For this review, take the finished solid that the model builds, in its own axes (mm). A direction names the side the tool comes from. Coordinates: 2 decimals unless noted, no trailing zeros. Write each loop counter-clockwise with the first axis right and the second up, starting at its lowest first coordinate (ties: lowest second). Pieces come first, ordered by that corner, then holes.
```python
from build123d import *

# Parameters (mm, degrees)
SKETCH1_R           = 10.5
SKETCH1_R_2         = 8
BOSS_EXTRUDE1_DEPTH = 7


with BuildPart() as part:
    # Sketch1 → Boss-Extrude1 (new body)
    with BuildSketch(Plane.XY):
        with BuildLine():
            Line((25.403411844, 18), (40.04634859, 43.362310416))
            ThreePointArc((40.04634859, 43.362310416), (40.729032534, 47.562011618), (38.455388874, 51.158411493))
            ThreePointArc((38.455388874, 51.158411493), (-35.819868425, 53.037128749), (-61.819252882, -16.564418887))
            Line((-61.819252882, -16.564418887), (-60.007519567, -23.325899671))
            ThreePointArc((-60.007519567, -23.325899671), (-57.211964609, -26.969137823), (-52.659050338, -27.568540358))
            Line((-52.659050338, -27.568540358), (-10.79860525, -16.352067901))
            ThreePointArc((-10.79860525, -16.352067901), (-8.844993295, -16.161017697), (-6.934268235, -16.610717144))
            ThreePointArc((-6.934268235, -16.610717144), (4.455015534, -17.439978113), (14.051245496, -11.25))
            ThreePointArc((14.051245496, -11.25), (16.136917784, -9.591673087), (18.734993995, -9))
            Line((18.734993995, -9), (68.906523061, -9))
            ThreePointArc((68.906523061, -9), (71.299695166, -9.497934272), (73.295653135, -10.909090909))
            ThreePointArc((73.295653135, -10.909090909), (101, 0), (73.295653135, 10.909090909))
            ThreePointArc((73.295653135, 10.909090909), (71.299695166, 9.497934272), (68.906523061, 9))
            Line((68.906523061, 9), (30.599564267, 9))
            ThreePointArc((30.599564267, 9), (25.403411844, 12), (25.403411844, 18))
        make_face()
        Circle(SKETCH1_R, mode=Mode.SUBTRACT)
        with Locations((85, 0)):
            Circle(SKETCH1_R_2, mode=Mode.SUBTRACT)
        with BuildLine():
            Line((-22.446087833, -6.014411108), (-43.078559215, -11.542865153))
            ThreePointArc((-43.078559215, -11.542865153), (-47.971955445, -10.731402919), (-50.582336617, -6.513618221))
            ThreePointArc((-50.582336617, -6.513618221), (-31.046832879, 40.461020355), (19.383344125, 47.172936845))
            ThreePointArc((19.383344125, 47.172936845), (22.781794932, 43.559859246), (22.299103121, 38.623179569))
            Line((22.299103121, 38.623179569), (11.618950039, 20.124611797))
            ThreePointArc((11.618950039, 20.124611797), (8.69359949, 17.570923037), (4.817098212, 17.343458848))
            ThreePointArc((4.817098212, 17.343458848), (-10.957705722, 14.280360125), (-17.999251578, -0.164142113))
            ThreePointArc((-17.999251578, -0.164142113), (-19.222277472, -3.849682749), (-22.446087833, -6.014411108))
        make_face(mode=Mode.SUBTRACT)
    extrude(amount=BOSS_EXTRUDE1_DEPTH)


solid = part.part
```
1) Consider section D-D (z = 4.5). Give the boundary of the cut face in (x, y) (3 decimals), then the cut area to 3 significant figures.
2) Tool access review of faces 1 (the face through (50, 9, 3)), 2 (the face through (71.3, -9.5, 3.5)), 3 (the face through (17, 19, 0)): name each direction out of +Z, -Z, +X, -X, +Y, -Y from which nothing blocks a thin tool from reaching the whole face with its end or side.
3) The part is to be moulded in two halves that separate along X. For faces 4 (the face through (-47.91, -10.77, 3.45)), 5 (the face through (-34.895, 53.65, 3.451)), 6 (the face through (40.74, 47.5, 3.45)), say which applies: pulls with the +X half, pulls with the -X half, needs draft (parallel to the pull), parting line crosses it, or undercut.
4) Clearance check with flat-ended pins moving along their axes: P1, Ø4, axis at y = 4, z = 5, coming from the +X side; P2, Ø10, axis at x = -1, y = -14.5, coming from the -Z side; P3, Ø3.5, axis at x = 53, z = 2.5, coming from the +Y side; P4, Ø3.5, axis at x = 53.5, z = 3, coming from the -Y side. State where each tip first meets the part, or that it passes through.
5) Consider section B-B (x = 0). Give the boundary of the cut face in (y, z).
6) Consider section A-A (x = 85). Give the boundary of the cut face in (y, z).
7) Consider section C-C (y = 41.5). Give the boundary of the cut face in (x, z), then the cut area to 3 significant figures.
8) For L1, parallel to Y at x = 0, z = 1.5; L2, parallel to Y at x = -3.5, z = 5.75; L3, parallel to Y at x = 85, z = 5, list the stretches that pass through material, from the lowest coordinate up.
Results:
1. outline: (-61.819, -16.564) - (-60.008, -23.326) arc R6 ccw to (-52.659, -27.569) - (-10.799, -16.352) arc R6 cw to (-6.934, -16.611) arc R18 ccw to (14.051, -11.25) arc R6 cw to (18.735, -9) - (68.907, -9) arc R6 cw to (73.296, -10.909) arc R16 ccw (long way) to (73.296, 10.909) arc R6 cw to (68.907, 9) - (30.6, 9) arc R6 cw to (25.403, 18) - (40.046, 43.362) arc R6 ccw to (38.455, 51.158) arc R64 ccw to start; hole (-50.582, -6.514) arc R6 ccw to (-43.079, -11.543) - (-22.446, -6.014) arc R6 ccw to (-17.999, -0.164) arc R18 cw to (4.817, 17.343) arc R6 ccw to (11.619, 20.125) - (22.299, 38.623) arc R6 ccw to (19.383, 47.173) arc R51 ccw to start; hole circle Ø21 at (0, 0); hole circle Ø16 at (85, 0)
1. area: 5,250 mm2
2. face 1: +Z, -Z
2. face 2: +Z, -Z, -Y
2. face 3: -Z, +X, -X, +Y, -Y
3. face 4: undercut
3. face 5: parting line crosses it
3. face 6: pulls with the +X half
4. P1: stops at x = 100.87
4. P2: stops at z = 0
4. P3: stops at y = 9
4. P4: stops at y = -9
5. outline: (-18, 0) - (-10.5, 0) - (-10.5, 7) - (-18, 7) - close; (10.5, 0) - (18, 0) - (18, 7) - (10.5, 7) - close; (51, 0) - (64, 0) - (64, 7) - (51, 7) - close
6. outline: (-16, 0) - (-8, 0) - (-8, 7) - (-16, 7) - close; (8, 0) - (16, 0) - (16, 7) - (8, 7) - close
7. outline: (-48.72, 0) - (-29.64, 0) - (-29.64, 7) - (-48.72, 7) - close; (23.1, 0) - (38.97, 0) - (38.97, 7) - (23.1, 7) - close
7. area: 245 mm2
8. L1: y = -18 to -10.5, 10.5 to 18, 51 to 64
8. L2: y = -17.66 to -9.9, 9.9 to 17.66, 50.88 to 63.9
8. L3: y = -16 to -8, 8 to 16
